Geometry check sheet. Reference: the model listing, model coordinates, mm. Face numbers are marked on the shaded views. A direction names the side the tool comes from. Coordinates: 2 decimals unless noted, no trailing zeros. Order: outer loops, then holes, each group sorted by start corner. A loop starts at its lowest first (then second) coordinate and runs counter-clockwise, first axis right, second up. Notation, with made-up numbers: M 60.25,15.5 L 72.25,15.5 A3 cw 72.25,20.5 Z; hole C 45.5,-28.75 d11. An arc over 180 degrees is marked long. One line per item, written item: value. Start each with the question number.
1) Draft check along Y on the marked faces 6, 7 and 8. Enter one of: pulls with the +Y half, pulls with the -Y half, needs draft (parallel to the pull), parting line crosses it, or undercut.
2) Sectioned sample at A-A, the plane x = -14. Enter the section's corners in (y, z).
3) Go/stop test with flat-tipped pins: P1, Ø4, axis at x = -9, y = -29.5, coming from the -Z side; P2, Ø5.5, axis at x = 3.5, z = 11, coming from the +Y side; P3, Ø5.5, axis at x = 3.5, y = -3, coming from the -Z side. Record where each tip stops, or that it passes through.
4) Sectioned sample at C-C, the plane y = -22. Enter the section's corners in (x, z), then the cut area to 3 significant figures.
5) Sectioned sample at B-B, the plane z = 11. Enter the section's corners in (x, y), then the cut area to 3 significant figures.
6) Sectioned sample at D-D, the plane z = 0. Enter the section's corners in (x, y).
7) Access from +Z, -Z, +X, -X, +Y, -Y to the whole of each face (thin tool, end or side, straight path). Record for the marked faces 1, 2, 3, 4 and 5.
8) Thickness scan on L1, parallel to Y at x = 2.75, z = 10; L2, parallel to Y at x = -5, z = 21.85; L3, parallel to Y at x = 3.75, z = 0. Record the ranges inside material, lowest first. Write a range as from..to.
```python
from build123d import *

# Parameters (mm, degrees)
SKETCH_1_R                = 4
EXTRUDE_1_DEPTH           = 5
EXTRUDE_2_DEPTH           = 10
FILLET_1_R                = 10
EXTRUDE_3_DEPTH           = 7
EXTRUDE_3_DEPTH_BACK      = 3
SKETCH_7_W                = 8
SKETCH_7_H                = 5
HOLE_WIZARD_1_D           = 3.6
HOLE_WIZARD_1_CSINK_D     = 6.6
HOLE_WIZARD_1_CSINK_ANGLE = 90
FILLET_2_R                = 2
FILLET_3_R                = 3
MM_TRANSITIONAL_1_D       = 3
SKETCH_10_W               = 2
SKETCH_10_H               = 5
CUT_EXTRUDE_1_DEPTH       = 48.143222787
SKETCH_11_W               = 11.5
SKETCH_11_H               = 5
EXTRUDE_4_DEPTH           = 10
HOLE_WIZARD_2_D           = 3.6
HOLE_WIZARD_2_CSINK_D     = 6.6
HOLE_WIZARD_2_CSINK_ANGLE = 90
CUT_EXTRUDE_2_DEPTH       = 51.224331302
FILLET_5_R                = 1
FILLET_6_R                = 2
SKETCH_13_W               = 3.5
SKETCH_13_H               = 5
CUT_EXTRUDE_3_DEPTH       = 0.5


with BuildPart() as part:
    # 草图1 → 凸台-拉伸1 (new body)
    with BuildSketch(Plane(origin=(0, 0, 0), x_dir=(0, 0, -1), z_dir=(1, 0, 0))):
        Polygon((-23.41, -33), (-0.742923434, -33), (-0.742923434, -39.679407187), (15.257076566, -39.679407187), (15.257076566, -30.774808421), (6.3745949, 8), (-23.41, 8), align=None)
        Circle(SKETCH_1_R, mode=Mode.SUBTRACT)
        with Locations((7.257076566, -31.679407187)):
            Circle(SKETCH_1_R, mode=Mode.SUBTRACT)
    extrude(amount=EXTRUDE_1_DEPTH)

    # 草图2 → 凸台-拉伸2 (add)
    with BuildSketch(Plane.ZY):
        Polygon((23.41, -15), (23.41, -33), (11.91, -33), (11.91, -28), (18.41, -28), (18.41, -15), align=None)
    extrude(amount=EXTRUDE_2_DEPTH)

    # 圆角1
    fillet_1_edges = [part.edges().sort_by_distance(p)[0] for p in [
        (2.5, 8, -6.3745949),
        (2.5, -30.774808421, -15.257076566),
    ]]
    fillet(fillet_1_edges, radius=FILLET_1_R)

    # 草图7 → 凸台-拉伸3 (add, two sides: drawn at the far end of the back side and taken through both)
    with BuildSketch(Plane(origin=(0, 8, 0), x_dir=(1, 0, 0), z_dir=(0, 1, 0)).offset(-EXTRUDE_3_DEPTH_BACK)):
        with Locations((1, -20.91)):
            Rectangle(SKETCH_7_W, SKETCH_7_H)
    extrude(amount=EXTRUDE_3_DEPTH + EXTRUDE_3_DEPTH_BACK)

    # 打孔尺寸(%根据十字)槽半沉头木螺钉的类型1 (through all)
    with Locations(Plane(origin=(0, 0, 18.41), x_dir=(-1, 0, 0), z_dir=(0, 0, -1))):
        with Locations((5, -22)):
            CounterSinkHole(HOLE_WIZARD_1_D / 2, HOLE_WIZARD_1_CSINK_D / 2, counter_sink_angle=HOLE_WIZARD_1_CSINK_ANGLE)

    # 圆角2
    fillet_2_edges = [part.edges().sort_by_distance(p)[0] for p in [
        (2.5, -39.679407187, 0.742923434),
        (2.5, -39.679407187, -15.257076566),
        (-3, 5, 20.91),
        (5, 15, 20.91),
        (-3, 15, 20.91),
    ]]
    fillet(fillet_2_edges, radius=FILLET_2_R)

    # 圆角3
    # the kernel refuses this fillet: 3 mm, written as the material it adds along each edge
    with BuildSketch(Plane(origin=(0, 5, 23.41), x_dir=(0, -1, 0), z_dir=(0, 0, -1))) as fillet_3_piece_1:
        with BuildLine():
            CenterArc((2.582575695, 3), FILLET_3_R, 203.578178478, 66.421821522)
            Line((-0.166969722, 1.8), (-0.441924264, 1.68))
            ThreePointArc((-0.441924264, 1.68), (-0.3, 1), (-0.3, 0))
            Line((-0.3, 0), (0, -0.3))
            Line((0, -0.3), (2.582575695, -0.3))
            Line((2.582575695, -0.3), (2.582575695, 0))
        make_face()
    extrude(amount=5)

    # 大小mm Transitional 暗销孔1 (through all)
    with Locations(Plane(origin=(0, 0, 18.41), x_dir=(-1, 0, 0), z_dir=(0, 0, -1))):
        with Locations((-0.78249385, 9.508910889)):
            Hole(MM_TRANSITIONAL_1_D / 2)

    # 草图10 → 切除-拉伸1 (cut, through all)
    with BuildSketch(Plane.ZY):
        with Locations((22.41, -0.082575695)):
            Rectangle(SKETCH_10_W, SKETCH_10_H)
        with Locations((22.41, -9.082575695)):
            Rectangle(SKETCH_10_W, SKETCH_10_H)
    extrude(amount=-CUT_EXTRUDE_1_DEPTH, mode=Mode.SUBTRACT)

    # 草图11 → 凸台-拉伸4 (add)
    with BuildSketch(Plane.ZY.offset(10)):
        with Locations((17.66, -30.5)):
            Rectangle(SKETCH_11_W, SKETCH_11_H)
    extrude(amount=EXTRUDE_4_DEPTH)

    # 打孔尺寸(%根据十字)槽半沉头木螺钉的类型2 (through all)
    with Locations(Plane(origin=(0, -28, 0), x_dir=(1, 0, 0), z_dir=(0, 1, 0))):
        with Locations((-14, -17.41)):
            CounterSinkHole(HOLE_WIZARD_2_D / 2, HOLE_WIZARD_2_CSINK_D / 2, counter_sink_angle=HOLE_WIZARD_2_CSINK_ANGLE)

    # 草图12 → 切除-拉伸2 (cut, through all)
    with BuildSketch(Plane.ZY):
        with BuildLine():
            Line((7.5, 0), (13.41, 0))
            Line((13.41, 0), (13.41, -10))
            Line((13.41, -10), (-2.290786732, -10))
            Line((-2.290786732, -10), (-1.674709977, -7.310632428))
            ThreePointArc((-1.674709977, -7.310632428), (4.673846124, -5.865591395), (7.5, 0))
        make_face()
        Polygon((-5.538986517, -24.179407187), (13.41, -24.179407187), (13.41, -15), (-3.436180098, -15), align=None)
    extrude(amount=-CUT_EXTRUDE_2_DEPTH, mode=Mode.SUBTRACT)

    # 圆角5
    fillet_5_edges = [part.edges().sort_by_distance(p)[0] for p in [
        (2.5, 0, 13.41),
        (2.5, -10, 13.41),
        (2.5, -10, -2.290786732),
        (2.5, -24.179407187, -5.538986517),
        (2.5, -15, -3.436180098),
        (2.5, -15, 13.41),
        (2.5, -24.179407187, 13.41),
    ]]
    fillet(fillet_5_edges, radius=FILLET_5_R)

    # 圆角6
    fillet_6_edges = [part.edges().sort_by_distance(p)[0] for p in [
        (-20, -30.5, 11.91),
    ]]
    fillet(fillet_6_edges, radius=FILLET_6_R)

    # 草图13 → 切除-拉伸3 (cut)
    with BuildSketch(Plane.XZ.offset(33)):
        with Locations((-18.25, 14.41)):
            Rectangle(SKETCH_13_W, SKETCH_13_H)
    extrude(amount=-CUT_EXTRUDE_3_DEPTH, mode=Mode.SUBTRACT)


solid = part.part
```
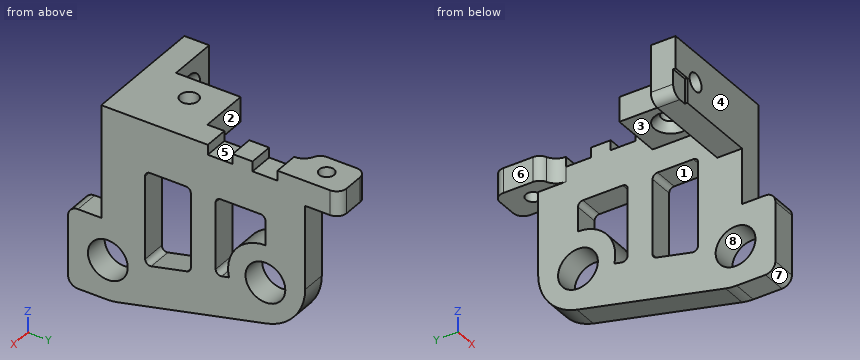
Final values:
1. face 6: needs draft
1. face 7: pulls with the -Y half
1. face 8: undercut
2. outline: M -33,11.91 L -28,11.91 L -28,14.11 L -29.5,15.61 L -33,15.61 Z; M -33,19.21 L -29.5,19.21 L -28,20.71 L -28,23.41 L -33,23.41 Z
3. P1: stops at z = 11.91
3. P2: stops at y = 8
3. P3: stops at z = -9.52
4. outline: M -10,18.41 L -8.3,18.41 L -6.8,19.91 L -6.8,23.41 L -10,23.41 Z; M -3.2,19.91 L -1.7,18.41 L 0,18.41 L 0,13.41 L 5,13.41 L 5,23.41 L -3.2,23.41 Z; M 0,-13.25 L 5,-13.25 L 5,-5.04 L 0,-5.04 Z
4. area: 121 mm^2
5. outline: M 0,-33 L 5,-33 L 5,-24.18 L 0,-24.18 Z; M 0,-15 L 5,-15 L 5,-10 L 0,-10 Z; M 0,0 L 5,0 L 5,8 L 0,8 Z
5. area: 109 mm^2
6. outline: M 0,-39.23 L 5,-39.23 L 5,-24.18 L 0,-24.18 Z; M 0,-15 L 5,-15 L 5,-10 L 0,-10 Z; M 0,-7.5 L 5,-7.5 L 5,-4 L 0,-4 Z; M 0,4 L 5,4 L 5,7.87 L 0,7.87 Z
7. face 1: +X, -X
7. face 2: +Z, -Z, -X
7. face 3: -Z, -X, +Y
7. face 4: +Z, +X, -X, -Y
7. face 5: +Z, +X, -X
8. L1: y = -33..-24.18, -15..-10, 0..8
8. L2: y = -33..-23.8, -20.2..-15
8. L3: y = -39.23..-24.18, -15..-10, -7.5..-4, 4..7.87
